Geometry check sheet. Reference: the model listing, model coordinates, mm. Round coordinates to 2 decimals unless told otherwise and drop trailing zeros. Write each loop counter-clockwise with the first axis right and the second up, starting at its lowest first coordinate (ties: lowest second). Pieces come first, ordered by that corner, then holes. Notation, with made-up numbers: (22, 3.25) -> (66, 3.25) arc R26 cw to (66, 17.25) -> close; hole circle Ø7 at (8.5, -9). An arc over 180 degrees is marked (long way). Use a Markdown table: item, result.
```python
from build123d import *

# Parameters (mm, degrees)
SKETCH_W   = 381
SKETCH_H   = 495
SKETCH_R   = 3
SKETCH_R_2 = 4.2
SKETCH_R_3 = 2.2
SKETCH_R_4 = 2.25
SKETCH_R_5 = 1.8
SKETCH_R_6 = 2.4
SKETCH_W_2 = 255
SKETCH_H_2 = 277.586411
SKETCH_W_3 = 81
SKETCH_H_3 = 59
PAD_DEPTH  = 8
FILLET_R   = 20


with BuildPart() as part:
    # Sketch → Pad (new body)
    with BuildSketch(Plane.XY):
        with Locations((-190.5, 247.5)):
            Rectangle(SKETCH_W, SKETCH_H)
        with Locations((-348.25, 412)):
            Circle(SKETCH_R, mode=Mode.SUBTRACT)
        with Locations((-315.75, 412)):
            Circle(SKETCH_R, mode=Mode.SUBTRACT)
        with Locations((-332, 412)):
            Circle(SKETCH_R_2, mode=Mode.SUBTRACT)
        with Locations((-63.25, 412)):
            Circle(SKETCH_R, mode=Mode.SUBTRACT)
        with Locations((-30.75, 412)):
            Circle(SKETCH_R, mode=Mode.SUBTRACT)
        with Locations((-47, 412)):
            Circle(SKETCH_R_2, mode=Mode.SUBTRACT)
        with Locations((-330, 452)):
            Circle(SKETCH_R_3, mode=Mode.SUBTRACT)
        with Locations((-290, 452)):
            Circle(SKETCH_R_3, mode=Mode.SUBTRACT)
        with Locations((-61, 452)):
            Circle(SKETCH_R_3, mode=Mode.SUBTRACT)
        with Locations((-21, 452)):
            Circle(SKETCH_R_3, mode=Mode.SUBTRACT)
        with Locations((-21, 482)):
            Circle(SKETCH_R_4, mode=Mode.SUBTRACT)
        with Locations((-360, 482)):
            Circle(SKETCH_R_4, mode=Mode.SUBTRACT)
        with Locations((-21, 13)):
            Circle(SKETCH_R_4, mode=Mode.SUBTRACT)
        with Locations((-360, 13)):
            Circle(SKETCH_R_4, mode=Mode.SUBTRACT)
        with Locations((-377, 96)):
            Circle(SKETCH_R_5, mode=Mode.SUBTRACT)
        with Locations((-275, 96)):
            Circle(SKETCH_R_5, mode=Mode.SUBTRACT)
        with Locations((-275, 39)):
            Circle(SKETCH_R_5, mode=Mode.SUBTRACT)
        with Locations((-377, 39)):
            Circle(SKETCH_R_5, mode=Mode.SUBTRACT)
        with Locations((-210.5, 13)):
            Circle(SKETCH_R_6, mode=Mode.SUBTRACT)
        with Locations((-170.5, 13)):
            Circle(SKETCH_R_6, mode=Mode.SUBTRACT)
        with Locations((-189.5, 248.793205)):
            Rectangle(SKETCH_W_2, SKETCH_H_2, mode=Mode.SUBTRACT)
        with Locations((-326, 67.5)):
            Rectangle(SKETCH_W_3, SKETCH_H_3, mode=Mode.SUBTRACT)
        with BuildLine():
            Line((-337.5, 31), (-315.5, 31))
            Line((-315.5, 31), (-315.5, 21.5))
            Line((-315.5, 21.5), (-313, 21.5))
            ThreePointArc((-313, 17.5), (-311, 19.5), (-313, 21.5))
            Line((-315.5, 17.5), (-313, 17.5))
            Line((-315.5, 17.5), (-315.5, 8))
            Line((-315.5, 8), (-337.5, 8))
            Line((-337.5, 8), (-337.5, 17.5))
            Line((-340, 17.5), (-337.5, 17.5))
            ThreePointArc((-340, 21.5), (-342, 19.5), (-340, 17.5))
            Line((-340, 21.5), (-337.5, 21.5))
            Line((-337.5, 21.5), (-337.5, 31))
        make_face(mode=Mode.SUBTRACT)
        with BuildLine():
            Line((-295.5, 27), (-273.5, 27))
            Line((-273.5, 27), (-273.5, 21.5))
            Line((-273.5, 21.5), (-271, 21.5))
            ThreePointArc((-271, 17.5), (-269, 19.5), (-271, 21.5))
            Line((-273.5, 17.5), (-271, 17.5))
            Line((-273.5, 17.5), (-273.5, 12))
            Line((-273.5, 12), (-295.5, 12))
            Line((-295.5, 12), (-295.5, 17.5))
            Line((-298, 17.5), (-295.5, 17.5))
            ThreePointArc((-298, 21.5), (-300, 19.5), (-298, 17.5))
            Line((-298, 21.5), (-295.5, 21.5))
            Line((-295.5, 21.5), (-295.5, 27))
        make_face(mode=Mode.SUBTRACT)
        with BuildLine():
            Line((-89, 58.5), (-66.5, 58.5))
            Line((-66.5, 64), (-66.5, 58.5))
            ThreePointArc((-62.5, 64), (-64.5, 66), (-66.5, 64))
            Line((-62.5, 64), (-62.5, 58.5))
            Line((-62.5, 58.5), (-40, 58.5))
            Line((-40, 58.5), (-40, 30))
            Line((-40, 30), (-62.5, 30))
            Line((-62.5, 30), (-62.5, 25))
            ThreePointArc((-66.5, 25), (-64.5, 23), (-62.5, 25))
            Line((-66.5, 30), (-66.5, 25))
            Line((-66.5, 30), (-89, 30))
            Line((-89, 30), (-89, 58.5))
        make_face(mode=Mode.SUBTRACT)
    extrude(amount=PAD_DEPTH)

    # Fillet
    fillet_edges = [part.edges().sort_by_distance(p)[0] for p in [
        (-317, 387.586411, 4),
        (-62, 387.586411, 4),
        (-62, 110, 4),
        (-317, 110, 4),
    ]]
    fillet(fillet_edges, radius=FILLET_R)


solid = part.part
```
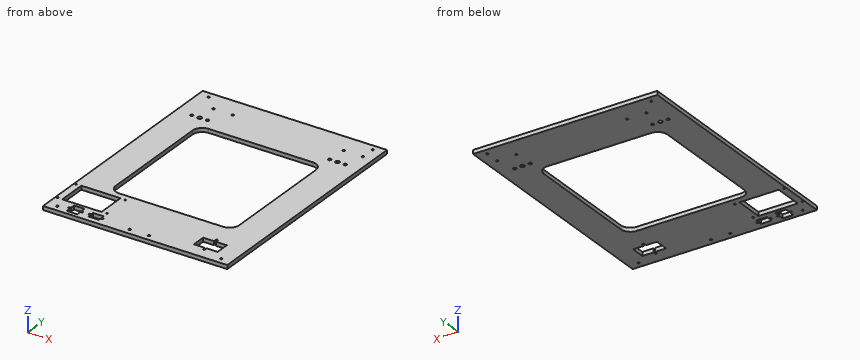
(1) Gauge pin test, flat end, axial feed: pin 1 Ø4 at (x, z) = (-341.5, 3) entering from -Y. Record the tip position at first contact, or that the pin passes through.
A:
| item | result |
|---|---|
| pin 1 | stops at y = 0 |
(2) Section check C-C on z = 4.5. State how many separate pieces and enclosed holes the cut face has, plus the area to 3 significant figures.
A:
| item | result |
|---|---|
| separate pieces | 1 |
| enclosed holes | 25 |
| area | 111,000 mm2 |
(3) Section check B-B on y = 318.5. Record the cut outline in (x, z).
A:
| item | result |
|---|---|
| outline | (-381, 0) -> (-317, 0) -> (-317, 8) -> (-381, 8) -> close; (-62, 0) -> (0, 0) -> (0, 8) -> (-62, 8) -> close |
(4) Thickness scan on line 1 (Y direction, x = -377, z = 2); line 2 (Y direction, x = -360, z = 6); line 3 (Y direction, x = -171, z = 1). Record the ranges inside material, lowest first.
A:
| item | result |
|---|---|
| line 1 | y = 0 to 37.2, 40.8 to 94.2, 97.8 to 495 |
| line 2 | y = 0 to 10.75, 15.25 to 38, 97 to 479.75, 484.25 to 495 |
| line 3 | y = 0 to 10.65, 15.35 to 110, 387.59 to 495 |
(5) Section check A-A on x = -179. Record the cut outline in (y, z).
A:
| item | result |
|---|---|
| outline | (0, 0) -> (110, 0) -> (110, 8) -> (0, 8) -> close; (387.59, 0) -> (495, 0) -> (495, 8) -> (387.59, 8) -> close |
